```python
from build123d import *

# Parameters (mm, degrees)
EXTRUDE_1_DEPTH     = 0.5
SKETCH_3_W          = 25
SKETCH_3_H          = 35
CUT_EXTRUDE_1_DEPTH = 114.058613257
SKETCH_4_W          = 10
SKETCH_4_H          = 35
CUT_EXTRUDE_2_DEPTH = 114.058613257
SKETCH_5_W          = 50
SKETCH_5_H          = 20
CUT_EXTRUDE_3_DEPTH = 114.058613257
SKETCH_6_W          = 10
SKETCH_6_H          = 20
CUT_EXTRUDE_4_DEPTH = 114.058613257
EXTRUDE_2_DEPTH     = 0.5
CUT_EXTRUDE_5_DEPTH = 119.289418767
FILLET_1_R          = 5
FILLET_2_R          = 20


with BuildPart() as part:
    # ｽｹｯﾁ1 → ﾎﾞｽ - 押し出し1 (new, symmetric)
    with BuildSketch(Plane(origin=(0, 0, 0), x_dir=(1, 0, 0), z_dir=(0, 1, 0))):
        with BuildLine():
            Line((62.68888804, 92.5), (-62.68888804, 92.5))
            add(Edge.make_bspline(
                [(-62.68888804, 92.5), (-67.396314277, 0), (-62.68888804, -92.5)],
                knots=[4.444925752, 4.444925752, 4.444925752, 4.979852209, 4.979852209, 4.979852209], degree=2, weights=[1, 0.964444431, 1]))
            Line((-62.68888804, -92.5), (62.68888804, -92.5))
            add(Edge.make_bspline(
                [(62.68888804, -92.5), (67.396314277, 0), (62.68888804, 92.5)],
                knots=[1.303333099, 1.303333099, 1.303333099, 1.838259555, 1.838259555, 1.838259555], degree=2, weights=[1, 0.964444431, 1]))
        make_face()
    extrude(amount=EXTRUDE_1_DEPTH, both=True)

    # ｽｹｯﾁ3 → ｶｯﾄ - 押し出し1 (cut, through all)
    with BuildSketch(Plane(origin=(0, 0.5, 0), x_dir=(1, 0, 0), z_dir=(0, 1, 0))):
        with Locations((-52.5, 75)):
            Rectangle(SKETCH_3_W, SKETCH_3_H)
    extrude(amount=-CUT_EXTRUDE_1_DEPTH, mode=Mode.SUBTRACT)

    # ｽｹｯﾁ4 → ｶｯﾄ - 押し出し2 (cut, through all)
    with BuildSketch(Plane(origin=(0, 0.5, 0), x_dir=(1, 0, 0), z_dir=(0, 1, 0))):
        with Locations((60, 75)):
            Rectangle(SKETCH_4_W, SKETCH_4_H)
    extrude(amount=-CUT_EXTRUDE_2_DEPTH, mode=Mode.SUBTRACT)

    # ｽｹｯﾁ5 → ｶｯﾄ - 押し出し3 (cut, through all)
    with BuildSketch(Plane(origin=(0, 0.5, 0), x_dir=(1, 0, 0), z_dir=(0, 1, 0))):
        with Locations((-40, -82.5)):
            Rectangle(SKETCH_5_W, SKETCH_5_H)
    extrude(amount=-CUT_EXTRUDE_3_DEPTH, mode=Mode.SUBTRACT)

    # ｽｹｯﾁ6 → ｶｯﾄ - 押し出し4 (cut, through all)
    with BuildSketch(Plane(origin=(0, 0.5, 0), x_dir=(1, 0, 0), z_dir=(0, 1, 0))):
        with Locations((60, -82.5)):
            Rectangle(SKETCH_6_W, SKETCH_6_H)
    extrude(amount=-CUT_EXTRUDE_4_DEPTH, mode=Mode.SUBTRACT)

    # ｽｹｯﾁ7 → ﾎﾞｽ - 押し出し2 (add, symmetric)
    with BuildSketch(Plane(origin=(0, 0, 0), x_dir=(1, 0, 0), z_dir=(0, 1, 0))):
        with BuildLine():
            Line((-15, -92.5), (55, -92.5))
            ThreePointArc((55, -92.5), (20, -98.825030024), (-15, -92.5))
        make_face()
    extrude(amount=EXTRUDE_2_DEPTH, both=True)

    # ｽｹｯﾁ8 → ｶｯﾄ - 押し出し5 (cut, through all)
    with BuildSketch(Plane(origin=(0, 0.5, 0), x_dir=(1, 0, 0), z_dir=(0, 1, 0))):
        with BuildLine():
            ThreePointArc((-40, 67.5), (-32.677669545, 85.177669514), (-15.000000044, 92.5))
            Line((-15.000000044, 92.5), (-40, 92.5))
            Line((-40, 92.5), (-40, 67.5))
        make_face()
        with BuildLine():
            Line((55, 67.5), (55, 92.5))
            Line((55, 92.5), (30, 92.5))
            ThreePointArc((30, 92.5), (47.67766953, 85.17766953), (55, 67.5))
        make_face()
    extrude(amount=-CUT_EXTRUDE_5_DEPTH, mode=Mode.SUBTRACT)

    # ﾌｨﾚｯﾄ1
    fillet_1_edges = [part.edges().sort_by_distance(p)[0] for p in [
        (-64.116831739, -0.25, -57.5),
        (-63.590195865, -0.25, 72.5),
        (63.590195865, -0.2499997, 72.5),
        (64.116831739, -0.25, -57.5),
    ]]
    fillet(fillet_1_edges, radius=FILLET_1_R)

    # ﾌｨﾚｯﾄ2
    fillet_2_edges = [part.edges().sort_by_distance(p)[0] for p in [
        (-15, 0, 92.5),
        (55, 0, 92.5),
    ]]
    fillet(fillet_2_edges, radius=FILLET_2_R)


solid = part.part
```
The model under review builds one solid part; all positions refer to its coordinate system, in mm. Round coordinates to 2 decimals unless told otherwise and drop trailing zeros. Loops run counter-clockwise (first coordinate to the right, second up) from the corner with the lowest first, then second, coordinate; pieces in that order, holes last. Notation, with made-up numbers: (57.5, 40) - (79.5, 40) arc R17 ccw to (79.5, 62) - close; hole circle Ø5 at (-28.5, -2.75). An arc over 180 degrees is marked (long way). Write each question's results on one line, items separated by ' | '. Start each with the question number.
Q1. Wall thickness on line 1 along X through (y, z) = (0.05, -51.5); line 2 along Z through (x, y) = (-51.5, 0.4); line 3 along Z through (x, y) = (-16, -0.3): over which ranges is each line inside the solid? List them lowest first. Write a range as [from, to].
Q2. Take a section at A-A on z = -59.5. Give the boundary of the cut face in (x, y).
Q3. Insertion check: P1, Ø0.5, axis at y = 0, z = -63, coming from the +X side; P2, Ø0.5, axis at x = 56, y = 0, coming from the -Z side; P3, Ø0.5, axis at y = 0, z = 74, coming from the -X side. Each pin has a flat end and moves straight along its axis. Give the tip position at first contact, or say it passes through.
Q4. Take a section at B-B on x = -26. Give the boundary of the cut face in (y, z).
Data:
1) line 1: x = [-64.29, 64.29] | line 2: z = [-57.5, 72.5] | line 3: z = [-92.48, 72.5]
2) outline: (-40, -0.5) - (55, -0.5) - (55, 0.5) - (-40, 0.5) - close
3) P1: stops at x = 55 | P2: stops at z = -57.5 | P3: stops at x = -15
4) outline: (-0.5, -89.95) - (0.5, -89.95) - (0.5, 72.5) - (-0.5, 72.5) - close
